```python
from build123d import *
from build123d.topology import SkipClean

# Parameters (mm, degrees)
SKETCH1_W                        = 150
SKETCH1_H                        = 100
BOSS_EXTRUDE1_DEPTH              = 12
SKETCH2_W                        = 8
SKETCH2_H                        = 44
BOSS_EXTRUDE2_DEPTH              = 65
FILLET1_R                        = 6
CUT_EXTRUDE1_DEPTH               = 179.339563754
F_5_0_5_DIAMETER_HOLE1_D         = 5
M12X1_5_TAPPED_HOLE1_D           = 10.5
M12X1_5_TAPPED_HOLE1_CSINK_D     = 12.05
M12X1_5_TAPPED_HOLE1_CSINK_ANGLE = 90
SKETCH8_R                        = 7.5
BOSS_EXTRUDE3_DEPTH              = 25
BOSS_EXTRUDE4_DEPTH              = 12
CUT_EXTRUDE2_DEPTH               = 214.848661441
CUT_EXTRUDE2_DEPTH_BACK          = 214.848661441
SKETCH10_R                       = 6
REVOLVE1_ANGLE                   = 180
SKETCH12_W                       = 43
SKETCH12_H                       = 11
BOSS_EXTRUDE5_DEPTH              = 18
FILLET2_R                        = 6


with BuildPart() as part:
    # Sketch1 → Boss-Extrude1 (new body)
    with BuildSketch(Plane(origin=(0, 0, 0), x_dir=(1, 0, 0), z_dir=(0, 1, 0))):
        with Locations((75, 50)):
            Rectangle(SKETCH1_W, SKETCH1_H)
    extrude(amount=BOSS_EXTRUDE1_DEPTH)

    # Sketch2 → Boss-Extrude2 (add)
    with BuildSketch(Plane(origin=(0, 12, 0), x_dir=(1, 0, 0), z_dir=(0, 1, 0))):
        with Locations((20, 22)):
            Rectangle(SKETCH2_W, SKETCH2_H)
    extrude(amount=BOSS_EXTRUDE2_DEPTH)

    # Fillet1
    fillet1_edges = [part.edges().sort_by_distance(p)[0] for p in [
        (16, 12, -22),
        (24, 12, -22),
        (20, 12, -44),
    ]]
    fillet(fillet1_edges, radius=FILLET1_R)

    # Sketch3 → Cut-Extrude1 (cut, through all)
    with BuildSketch(Plane(origin=(24, 0, 0), x_dir=(0, 0, -1), z_dir=(1, 0, 0))):
        with BuildLine():
            Line((44, 77), (29, 77))
            ThreePointArc((29, 77), (39.606601718, 72.606601718), (44, 62))
            Line((44, 62), (44, 77))
        make_face()
    extrude(amount=-CUT_EXTRUDE1_DEPTH, mode=Mode.SUBTRACT)

    # Ø5.0 (5) Diameter Hole1 (through all)
    with Locations(Plane(origin=(24, 0, 0), x_dir=(0, 0, -1), z_dir=(1, 0, 0))):
        with Locations((22, 60), (22, 35)):
            Hole(F_5_0_5_DIAMETER_HOLE1_D / 2)

    # M12x1.5 Tapped Hole1 (through all)
    with Locations(Plane(origin=(24, 0, 0), x_dir=(0, 0, -1), z_dir=(1, 0, 0))):
        with Locations((22, 47.5)):
            CounterSinkHole(M12X1_5_TAPPED_HOLE1_D / 2, M12X1_5_TAPPED_HOLE1_CSINK_D / 2, counter_sink_angle=M12X1_5_TAPPED_HOLE1_CSINK_ANGLE)

    # Sketch8 → Boss-Extrude3 (add)
    with BuildSketch(Plane(origin=(0, 12, 0), x_dir=(1, 0, 0), z_dir=(0, 1, 0))):
        with Locations(Location((55, 75, 0), (0, 0, 90))):
            Circle(SKETCH8_R)
    extrude(amount=BOSS_EXTRUDE3_DEPTH)

    # Sketch9 → Boss-Extrude4 (add)
    with BuildSketch(Plane(origin=(0, 12, 0), x_dir=(1, 0, 0), z_dir=(0, 1, 0))):
        with BuildLine():
            ThreePointArc((177.5, 0), (169.445436483, 19.445436483), (150, 27.5))
            Line((150, 27.5), (150, 0))
            Line((150, 0), (122.5, 0))
            ThreePointArc((122.5, 0), (150, -27.5), (177.5, 0))
        make_face()
        with BuildLine():
            Line((150, 0), (150, 27.5))
            ThreePointArc((150, 27.5), (130.554563517, 19.445436483), (122.5, 0))
            Line((122.5, 0), (150, 0))
        make_face()
    extrude(amount=-BOSS_EXTRUDE4_DEPTH)

    # Sketch10 → Cut-Extrude2 (cut, two sides: drawn at the far end of the back side and taken through both)
    with BuildSketch(Plane(origin=(0, 12, 0), x_dir=(1, 0, 0), z_dir=(0, 1, 0)).offset(-CUT_EXTRUDE2_DEPTH_BACK)):
        with Locations(Location((90, 60, 0), (0, 0, 270))):
            Circle(SKETCH10_R)
        with Locations(Location((110, 60, 0), (0, 0, 270))):
            Circle(SKETCH10_R)
        with Locations(Location((90, 40, 0), (0, 0, 270))):
            Circle(SKETCH10_R)
        with Locations(Location((110, 40, 0), (0, 0, 270))):
            Circle(SKETCH10_R)
        with Locations(Location((90, 25, 0), (0, 0, 270))):
            Circle(SKETCH10_R)
        with Locations(Location((110, 25, 0), (0, 0, 270))):
            Circle(SKETCH10_R)
    extrude(amount=CUT_EXTRUDE2_DEPTH + CUT_EXTRUDE2_DEPTH_BACK, mode=Mode.SUBTRACT)

    # Sketch11 → Revolve1 (revolve)
    with SkipClean():  # the faces are left unmerged after this step: merging them gives an invalid solid
        with BuildSketch(Plane(origin=(0, 37, 0), x_dir=(1, 0, 0), z_dir=(0, 1, 0))):
            with BuildLine():
                ThreePointArc((62.5, 75), (60.303300859, 80.303300859), (55, 82.5))
                Line((55, 82.5), (55, 67.5))
                ThreePointArc((55, 67.5), (60.303300859, 69.696699141), (62.5, 75))
            make_face()
            with BuildLine():
                Line((55, 67.5), (55, 82.5))
                ThreePointArc((55, 82.5), (47.5, 75), (55, 67.5))
            make_face()
        revolve(axis=Axis((55, 37, -82.5), (0, 0, 1)), revolution_arc=REVOLVE1_ANGLE)

    # Sketch12 → Boss-Extrude5 (add)
    with BuildSketch(Plane(origin=(0, 12, 0), x_dir=(1, 0, 0), z_dir=(0, 1, 0))):
        with Locations((103.5, 88.5)):
            Rectangle(SKETCH12_W, SKETCH12_H)
    extrude(amount=BOSS_EXTRUDE5_DEPTH)

    # Fillet2
    fillet2_edges = [part.edges().sort_by_distance(p)[0] for p in [
        (82, 12, -88.5),
        (103.5, 12, -83),
        (125, 12, -88.5),
        (103.5, 12, -94),
    ]]
    fillet(fillet2_edges, radius=FILLET2_R - 0.0001)  # a hair under: the kernel refuses the full size


solid = part.part
```
Can you work these out from the model? Positions are in its coordinate system, mm. A direction names the side the tool comes from. Give positions to 0.01 mm unless a question says otherwise; leave off trailing zeros. Loops run counter-clockwise (first coordinate to the right, second up) from the corner with the lowest first, then second, coordinate; pieces in that order, holes last. Notation, with made-up numbers: M 73,-38 L 90,-38 A8 ccw 90,-34 Z; hole C -38.75,-35 d3. An arc over 180 degrees is marked long. Answer in a Markdown table with one row per item.
1. Suppose I cut it at A-A on y = 60. Write out the boundary of the cut face in (x, z), plus the area to 3 significant figures.
Taken from the geometry:
| item | result |
|---|---|
| outline | M 16,-44 L 24,-44 L 24,-24.5 L 16,-24.5 Z; M 16,-19.5 L 24,-19.5 L 24,0 L 16,0 Z |
| area | 312 mm² |
2. Thinking about a two-plate mould opening in X: for faces 1 (the cylindrical face through (20.06, 72.72, -39.49)), 2 (the flat face through (150, 6, -63)), 3 (the cylindrical face through (95.95, 5.92, -25.78)), which applies, released by +X, released by -X, zero draft, split by the parting line, or undercut?
Taken from the geometry:
| item | result |
|---|---|
| face 1 | zero draft |
| face 2 | released by +X |
| face 3 | undercut |
3. Which directions (+Z, -Z, +X, -X, +Y, -Y) give clear straight access to the entire face, cutting with the end or side of a thin tool? Please do faces 4 (the cylindrical face through (52.747, 24.325, -82.154)), 5 (the flat face through (125, 24, -88)), 6 (the flat face through (103, 24, -83)).
Taken from the geometry:
| item | result |
|---|---|
| face 4 | +Y |
| face 5 | +Z, -Z, +X, +Y |
| face 6 | +Z, +X, -X, +Y |
4. Suppose I cut it at C-C on y = 26.5. Write out the boundary of the cut face in (x, z).
Taken from the geometry:
| item | result |
|---|---|
| outline | M 16,-44 L 24,-44 L 24,0 L 16,0 Z; C 55,-75 d15; M 82,-94 L 125,-94 L 125,-83 L 82,-83 Z |
5. If I drill on line 1 along X through (y, z) = (3.75, -40); line 2 along Y through (x, z) = (20.5, -22); line 3 along Z through (x, y) = (90, 3), over which ranges is the centre line in solid material (lowest first)?
Taken from the geometry:
| item | result |
|---|---|
| line 1 | x = 0 to 84, 96 to 104, 116 to 150 |
| line 2 | y = 0 to 32.5, 37.5 to 42.25, 52.75 to 57.5, 62.5 to 77 |
| line 3 | z = -100 to -66, -54 to -46, -34 to -31, -19 to 0 |
6. For pin 1 Ø9 at (x, y) = (22, 44.5) entering from -Z; pin 2 Ø6.5 at (y, z) = (35, -22) entering from -X; pin 3 Ø3.5 at (x, y) = (110.5, 25) entering from +Z, each with a flat end and sliding along its axis, tell me the tip position at first contact or that it passes through.
Taken from the geometry:
| item | result |
|---|---|
| pin 1 | stops at z = -44 |
| pin 2 | stops at x = 16 |
| pin 3 | stops at z = -83 |
7. Suppose I cut it at D-D on z = -40. Write out the boundary of the cut face in (x, y), plus the area to 3 significant figures.
Taken from the geometry:
| item | result |
|---|---|
| outline | M 0,0 L 84,0 L 84,12 L 30,12 A6 cw 24,18 L 24,72.2 L 16,72.2 L 16,18 A6 cw 10,12 L 0,12 Z; M 96,0 L 104,0 L 104,12 L 96,12 Z; M 116,0 L 150,0 L 150,12 L 116,12 Z |
| area | 2,010 mm² |
8. Suppose I cut it at B-B on x = 110. Count the separate pieces of the cut face and the enclosed holes in it, plus the area to 3 significant figures.
Taken from the geometry:
| item | result |
|---|---|
| separate pieces | 4 |
| enclosed holes | 0 |
| area | 981 mm² |
